Model file for the job. Use its own axes, mm. A direction names the side the tool comes from. Give positions to 0.01 mm unless a question says otherwise; leave off trailing zeros. Loops run counter-clockwise (first coordinate to the right, second up) from the corner with the lowest first, then second, coordinate; pieces in that order, holes last. Notation, with made-up numbers: M 41.25,81.5 L 84.25,81.5 A29 ccw 84.25,109.5 Z; hole C 83,-34 d11. An arc over 180 degrees is marked long. Answer in a Markdown table with one row per item.
```python
from build123d import *

# Parameters (mm, degrees)
F0_W      = 73.406
F0_H      = 15.875
F1_DEPTH  = 28.448
F2_W      = 35.052
F2_H      = 1.524
F3_DEPTH  = 28.575
F4_W      = 69.596
F4_H      = 6.35
F5_DEPTH  = 28.575
F7_DEPTH  = 4.826
F9_DEPTH  = 28.575
F11_DEPTH = 4.826
F13_DEPTH = 9.652
F15_DEPTH = 4.826
F17_DEPTH = 25.4
F18_W     = 11.049
F18_H     = 4.826
F19_DEPTH = 25.4
F21_DEPTH = 25.4


with BuildPart() as f1:
    # F0 (on Top) → F1 (new body)
    with BuildSketch(Plane.XY):
        Polygon((74.175101427, 28.0341930517), (-30.4715011545, 28.575), (-30.4715011545, 0), (42.9344988455, 0), (45.8496453135, 0), align=None)
        with Locations((6.2314988455, -7.9375)):
            Rectangle(F0_W, F0_H)
        Polygon((42.9344988455, -15.875), (-30.4715011545, -15.875), (-30.4715011545, -31.75), (-30.4715011545, -60.325), (74.175101427, -59.7841930517), (45.8496453135, -31.75), (42.9344988455, -31.75), align=None)
    extrude(amount=F1_DEPTH)

    # F2 (on face) → F3 (cut)
    with BuildSketch(Plane(origin=(0.3109336175, -60.1659183461, 0), x_dir=(0.9999866465, 0.005167867, 0), z_dir=(0.005167867, -0.9999866465, 0))):
        with Locations((56.3391541689, 27.686)):
            Rectangle(F2_W, F2_H)
        with Locations((56.3391541689, 0.762)):
            Rectangle(F2_W, F2_H)
    extrude(amount=-F3_DEPTH, mode=Mode.SUBTRACT)

    # F4 (on face) → F5 (cut)
    with BuildSketch(Plane(origin=(0.3109336175, -60.1659183461, 0), x_dir=(0.9999866465, 0.005167867, 0), z_dir=(0.005167867, -0.9999866465, 0))):
        with Locations((4.0151541689, 25.273)):
            Rectangle(F4_W, F4_H)
        Polygon((-24.4328458311, 11.176), (-30.7828458311, 11.176), (-30.7828458311, 0), (38.8131541689, 0), (38.8131541689, 6.35), (-24.4328458311, 6.35), align=None)
    extrude(amount=-F5_DEPTH, mode=Mode.SUBTRACT)

    # F6 (on face) → F7 (cut)
    with BuildSketch(Plane.XY.offset(26.924)):
        Polygon((42.9344988455, -31.75), (38.9777544369, -31.75), (39.0329974569, -42.4395711603), (56.5587634232, -42.3489991228), (45.8496453135, -31.75), align=None)
        Polygon((42.9344988455, -31.3702609057), (38.9758976941, -31.3907187032), (38.9777544369, -31.75), (42.9344988455, -31.75), align=None)
    extrude(amount=-F7_DEPTH, mode=Mode.SUBTRACT)

    # F8 (on face) → F9 (cut)
    with BuildSketch(Plane(origin=(0.1468560305, 28.4167662886, 0), x_dir=(-0.9999866465, 0.005167867, 0), z_dir=(0.005167867, 0.9999866465, 0))):
        Polygon((-48.6415103078, 28.448), (-74.0292339469, 28.448), (-74.0292339469, 26.924), (-48.6415103078, 26.924), (30.6187660531, 26.924), (30.6187660531, 28.448), align=None)
        Polygon((30.6187660531, 1.524), (-74.0292339469, 1.524), (-74.0292339469, 0), (-49.0522161126, 0), (30.6187660531, 0), align=None)
    extrude(amount=-F9_DEPTH, mode=Mode.SUBTRACT)

    # F10 (on face) → F11 (cut)
    with BuildSketch(Plane.XY.offset(26.924)):
        Polygon((39.1235694943, 10.6893371266), (39.1235694943, 28.2153371266), (-30.4715011545, 28.575), (-30.4715011545, -0.0003815818), (42.9344988455, -0.3797390943), (42.9344988455, 0), (45.8496453135, 0), (56.6500399995, 10.6893371266), align=None)
    extrude(amount=-F11_DEPTH, mode=Mode.SUBTRACT)

    # F12 (on face) → F13 (cut)
    with BuildSketch(Plane(origin=(0, 0, 1.524), x_dir=(1, 0, 0), z_dir=(0, 0, -1))):
        Polygon((-30.4715011545, 0.0003815818), (-30.4715011545, -28.575), (-24.1215859493, -28.5421840444), (-24.2692577495, 0.0324343789), align=None)
    extrude(amount=-F13_DEPTH, mode=Mode.SUBTRACT)

    # F14 (on face) → F15 (cut)
    with BuildSketch(Plane(origin=(0, 0, 1.524), x_dir=(1, 0, 0), z_dir=(0, 0, -1))):
        Polygon((38.9758976941, 0.3592812968), (-24.2692577495, 0.0324343789), (-24.1215859493, -28.5421840444), (39.1235694943, -28.2153371266), align=None)
    extrude(amount=-F15_DEPTH, mode=Mode.SUBTRACT)

    # F16 (on face) → F17 (cut)
    with BuildSketch(Plane(origin=(38.9767134639, -0.201429162, 0), x_dir=(-0.005167867, -0.9999866465, 0), z_dir=(-0.9999866465, 0.005167867, 0))):
        Polygon((0.1578542427, 6.35), (-0.2124354796, 6.35), (-10.8911457573, 6.35), (-10.8911457573, 1.524), (-0.2124354796, 1.524), (0.1578542427, 1.524), align=None)
    extrude(amount=-F17_DEPTH, mode=Mode.SUBTRACT)

    # F18 (on face) → F19 (cut)
    with BuildSketch(Plane(origin=(38.8126358769, 0.2005812195, 0), x_dir=(0.005167867, -0.9999866465, 0), z_dir=(-0.9999866465, -0.005167867, 0))):
        with Locations((37.1162217833, 3.937)):
            Rectangle(F18_W, F18_H)
    extrude(amount=-F19_DEPTH, mode=Mode.SUBTRACT)

    # F20 (on face) → F21 (cut)
    with BuildSketch(Plane.XY.offset(22.098)):
        with BuildLine():
            Line((0, -51.6199137252), (23.6292229191, -51.6253090635))
            ThreePointArc((23.6292229191, -51.6253090635), (29.2171637927, -45.9151668007), (23.384997691, -40.454704693))
            Line((23.384997691, -40.454704693), (0, -40.454704693))
            ThreePointArc((0, -40.454704693), (-5.8335011545, -46.0373092091), (0, -51.6199137252))
        make_face()
        with BuildLine():
            ThreePointArc((0, 19.870295307), (-5.8335011545, 14.2876907909), (0, 8.7050862748))
            Line((0, 8.7050862748), (23.384997691, 8.7050862748))
            ThreePointArc((23.384997691, 8.7050862748), (29.2171637927, 14.1655483825), (23.6292229191, 19.8756906452))
            Line((23.6292229191, 19.8756906452), (0, 19.870295307))
        make_face()
    extrude(amount=-F21_DEPTH, mode=Mode.SUBTRACT)


solid = f1.part
```
(1) Flat gauge pins, fed straight in: P1, Ø6, axis at y = 14, z = 9.5, coming from the -X side; P2, Ø8.5, axis at y = -22, z = 14, coming from the +X side; P3, Ø3, axis at x = 44.5, z = 14, coming from the +Y side; P4, Ø5, axis at x = -28.5, y = 9, coming from the -Z side. Where does each tip first touch, or does it go through?
Established:
| item | result |
|---|---|
| P1 | stops at x = -30.47 |
| P2 | stops at x = 42.93 |
| P3 | stops at y = 28.2 |
| P4 | stops at z = 11.18 |
(2) Saw through at A-A, the plane z = 19. Count the separate pieces of the cut face and the enclosed holes in it, and give its area (3 significant figures).
Established:
| item | result |
|---|---|
| separate pieces | 1 |
| enclosed holes | 2 |
| area | 6,730 mm2 |
(3) Saw through at C-C, the plane x = 52. Give the cut face in (y, z).
Established:
| item | result |
|---|---|
| outline | M -59.9,1.52 L -42.37,1.52 L -42.37,6.35 L -37.84,6.35 L -37.84,22.1 L -42.37,22.1 L -42.37,26.92 L -59.9,26.92 Z; M 6.09,6.35 L 10.62,6.35 L 10.62,1.52 L 28.15,1.52 L 28.15,26.92 L 10.69,26.92 L 10.69,22.1 L 6.09,22.1 Z |
(4) Which spindle directions (+Z, -Z, +X, -X, +Y, -Y) get a long thin tool onto all of the face, cutting with end or side? Do faces 3 (the flat face through (12, -40.455, 14)), 4 (the flat face through (44, 0, 14)), 5 (the flat face through (-30.472, -15, 14)). Say none if no direction does.
Established:
| item | result |
|---|---|
| face 3 | +Z, -Z |
| face 4 | +Z, -Z, +X |
| face 5 | +Z, -Z, -X, +Y, -Y |
(5) Saw through at D-D, the plane x = 21.5. Give the cut face in (y, z), and give its area (3 significant figures).
Established:
| item | result |
|---|---|
| outline | M -60.06,6.35 L -51.62,6.35 L -51.62,22.1 L -60.06,22.1 Z; M -40.45,6.35 L -31.48,6.35 L -31.48,0 L -0.27,0 L -0.27,6.35 L 8.71,6.35 L 8.71,22.1 L -0.27,22.1 L -0.27,28.45 L -31.48,28.45 L -31.48,22.1 L -40.45,22.1 Z; M 19.88,6.35 L 28.31,6.35 L 28.31,22.1 L 19.88,22.1 Z |
| area | 1,440 mm2 |
(6) Wall check: L1, parallel to Y at x = 20.5, z = 13.5; L2, parallel to X at y = -24, z = 25.5; L3, parallel to Z at x = 2, y = -55.5. Give the ranges that are in metal, low to high.
Established:
| item | result |
|---|---|
| L1 | y = -60.06 to -51.62, -40.45 to 8.71, 19.87 to 28.31 |
| L2 | x = -30.47 to 42.93 |
| L3 | z = 6.35 to 22.1 |
(7) Saw through at B-B, the plane y = 14.5. Give the cut face in (x, z).
Established:
| item | result |
|---|---|
| outline | M -30.47,11.18 L -24.19,11.18 L -24.19,6.35 L -5.83,6.35 L -5.83,22.1 L -30.47,22.1 Z; M 29.21,6.35 L 39.05,6.35 L 39.05,1.52 L 60.5,1.52 L 60.5,26.92 L 39.12,26.92 L 39.12,22.1 L 29.21,22.1 Z |
(8) Mould opens along Y. For faces 1 (the flat face through (6, -16, 28.448)), 2 (the flat face through (62.961, 16.936, 14.046)) say: pulls with the +Y half, pulls with the -Y half, needs draft (parallel to the pull), parting line crosses it, or undercut.
Established:
| item | result |
|---|---|
| face 1 | needs draft |
| face 2 | undercut |
